The model under review builds one solid part; all positions refer to its coordinate system, in mm. Face numbers are marked on the shaded views. A direction names the side the tool comes from. Round coordinates to 2 decimals unless told otherwise and drop trailing zeros. Order: outer loops, then holes, each group sorted by start corner. A loop starts at its lowest first (then second) coordinate and runs counter-clockwise, first axis right, second up. Notation, with made-up numbers: M 42.25,-19 L 72.25,-19 A27 cw 72.25,15 Z; hole C -22,58.25 d3. An arc over 180 degrees is marked long. Answer as a JSON object with one key per item and string values. Group by question number.
1. To check wall thickness, follow probe 1 along X at (y, z) = (17, 34); probe 2 along X at (y, z) = (25, 36); probe 3 along X at (y, z) = (6, 5). State the ranges of each line that lie inside material, in increasing order. Write a range as [from, to].
2. Mouldability with a two-part tool opening along Y and no side actions: class the marked faces 6, 7 and 8 as released by +Y, released by -Y, zero draft, split by the parting line, or undercut.
3. Clearance check with flat-ended pins moving along their axes: P1, Ø19, axis at y = 50, z = 21, coming from the -X side; P2, Ø1.5, axis at y = 31, z = 18.5, coming from the -X side; P3, Ø2.5, axis at x = 38.5, z = 19.5, coming from the -Y side; P4, Ø21, axis at x = 58, y = 16, coming from the +Z side. State where each tip first meets the part, or that it passes through.
4. Machinability: for the marked faces 1, 2, 3, 4 and 5, which of the approach directions +Z, -Z, +X, -X, +Y, -Y give a long, thin tool a straight path to every point of the face, cutting with its end or side? Answer none if there is none.
5. Add section A-A on z = 24. Give the number of separate pieces and of enclosed holes in the cut face, and give its area (3 significant figures).
6. Add section D-D on x = 37. State the section outline as (y, z) points, and give its area (3 significant figures).
7. Add section B-B on y = 57.5. State the section outline as (x, z) points, and give its area (3 significant figures).
```python
from build123d import *

# Parameters (mm, degrees)
SKETCH1_W               = 74
SKETCH1_H               = 32
SKETCH1_R               = 11.7
BOSS_EXTRUDE1_DEPTH     = 38.5
SKETCH2_R               = 1.575
SKETCH2_R_2             = 10.75
BOSS_EXTRUDE2_DEPTH     = 5
BOSS_EXTRUDE3_DEPTH     = 5
CUT_EXTRUDE1_DEPTH      = 112.012668196
CUT_EXTRUDE1_DEPTH_BACK = 112.012668196
SKETCH4_W               = 10
SKETCH4_H               = 25
SKETCH4_H_2             = 4.450035805
SKETCH5_R               = 2.15
CUT_EXTRUDE2_DEPTH      = 18
FILLET8_R               = 16
FILLET9_R               = 1.5
FILLET10_SIZE           = 2
CUT_EXTRUDE3_DEPTH      = 3


with BuildPart() as part:
    # Sketch1 → Boss-Extrude1 (new body)
    with BuildSketch(Plane.XY):
        with Locations((37, 16)):
            Rectangle(SKETCH1_W, SKETCH1_H)
        with Locations((16, 16)):
            Circle(SKETCH1_R, mode=Mode.SUBTRACT)
        with Locations((58, 16)):
            Circle(SKETCH1_R, mode=Mode.SUBTRACT)
    extrude(amount=BOSS_EXTRUDE1_DEPTH)

    # Sketch2 → Boss-Extrude2 (add)
    # profile 1 of 2: a face of its own
    with BuildSketch(Plane(origin=(74, 0, 0), x_dir=(0, 0, -1), z_dir=(1, 0, 0))):
        with BuildLine():
            Line((-38.5, 32), (0, 32))
            Line((0, 32), (0, 54))
            ThreePointArc((0, 54), (-19.25, 34.75), (-38.5, 54))
            Line((-38.5, 54), (-38.5, 32))
        make_face()
    # profile 2 of 2: a face of its own
    with BuildSketch(Plane(origin=(74, 0, 0), x_dir=(0, 0, -1), z_dir=(1, 0, 0))):
        with BuildLine():
            ThreePointArc((-38.5, 54), (-19.25, 34.75), (0, 54))
            ThreePointArc((0, 54), (-19.25, 73.25), (-38.5, 54))
        make_face()
        with Locations((-28.249026536, 43.275377796)):
            Circle(SKETCH2_R, mode=Mode.SUBTRACT)
        with Locations((-24.038282007, 67.155696691)):
            Circle(SKETCH2_R, mode=Mode.SUBTRACT)
        with Locations((-19.25, 54)):
            Circle(SKETCH2_R_2, mode=Mode.SUBTRACT)
        with Locations((-5.462691458, 51.568925513)):
            Circle(SKETCH2_R, mode=Mode.SUBTRACT)
    extrude(amount=-BOSS_EXTRUDE2_DEPTH)

    # Sketch3 → Boss-Extrude3 (add)
    with BuildSketch(Plane.ZY.offset(-69)):
        with BuildLine():
            Line((0, 43), (0, 32))
            Line((0, 32), (38.5, 32))
            Line((38.5, 32), (38.5, 43))
            Line((38.5, 43), (36.548843892, 43))
            ThreePointArc((36.548843892, 43), (19.25, 33.5), (1.951156108, 43))
            Line((1.951156108, 43), (0, 43))
        make_face()
    extrude(amount=BOSS_EXTRUDE3_DEPTH)

    # Sketch4 → Cut-Extrude1 (cut, two sides: drawn at the far end of the back side and taken through both)
    with BuildSketch(Plane(origin=(0, 0, 0), x_dir=(-1, 0, 0), z_dir=(0, 0, -1)).offset(-CUT_EXTRUDE1_DEPTH_BACK)):
        with Locations((-37, 23.950035805)):
            Rectangle(SKETCH4_W, SKETCH4_H)
        with Locations((-37, 34.225017902)):
            Rectangle(SKETCH4_W, SKETCH4_H_2)
    extrude(amount=CUT_EXTRUDE1_DEPTH + CUT_EXTRUDE1_DEPTH_BACK, mode=Mode.SUBTRACT)

    # Sketch5 → Cut-Extrude2 (cut)
    with BuildSketch(Plane(origin=(0, 11.450035805, 0), x_dir=(1, 0, 0), z_dir=(0, 1, 0))):
        with Locations(Location((37, -19.25, 0), (0, 0, 270))):
            Circle(SKETCH5_R)
    extrude(amount=-CUT_EXTRUDE2_DEPTH, mode=Mode.SUBTRACT)

    # Fillet8
    fillet8_edges = [part.edges().sort_by_distance(p)[0] for p in [
        (42, 32, 19.25),
        (32, 32, 19.25),
        (0, 32, 19.25),
        (0, 0, 19.25),
        (74, 0, 19.25),
    ]]
    fillet(fillet8_edges, radius=FILLET8_R - 0.0001)  # a hair under: the kernel refuses the full size

    # Fillet9
    fillet9_edges = [part.edges().sort_by_distance(p)[0] for p in [
        (66.5, 43, 36.548843892),
        (66.5, 43, 1.951156108),
        (64, 32, 19.25),
    ]]
    fillet(fillet9_edges, radius=FILLET9_R - 0.0001)  # a hair under: the kernel refuses the full size

    # Fillet10
    fillet10_edges = [part.edges().sort_by_distance(p)[0] for p in [
        (4.3, 16, 0),
        (4.3, 16, 38.5),
        (46.3, 16, 0),
        (46.3, 16, 38.5),
    ]]
    chamfer(fillet10_edges, length=FILLET10_SIZE)

    # Sketch6 → Cut-Extrude3 (cut)
    with BuildSketch(Plane.XZ):
        Polygon((39.110229916, 15.468871901), (41.329667947, 19.186948665), (39.219438031, 22.968076764), (34.889770084, 23.031128099), (32.670332053, 19.313051335), (34.780561969, 15.531923236), align=None)
    extrude(amount=-CUT_EXTRUDE3_DEPTH, mode=Mode.SUBTRACT)


solid = part.part
```
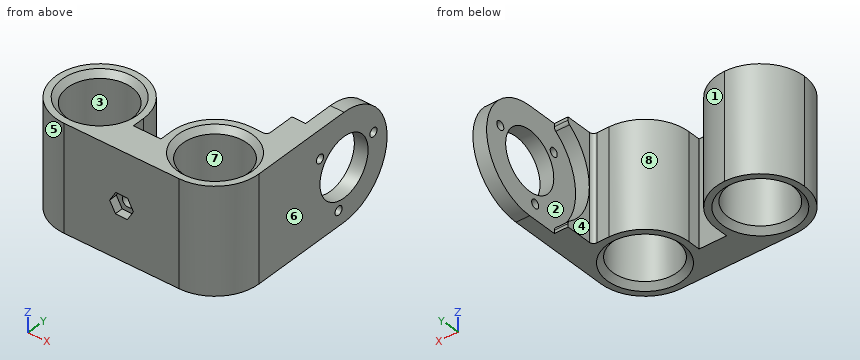
Recorded:
{
 "1": {"probe 1": "x = [0.03, 4.34], [27.66, 31.97], [42.03, 46.34], [69.66, 74]", "probe 2": "x = [2.77, 8.52], [23.48, 29.23], [44.77, 50.52], [65.48, 74]", "probe 3": "x = [3.51, 9.93], [22.07, 51.93], [64.07, 70.49]"},
 "2": {"face 6": "zero draft", "face 7": "undercut", "face 8": "released by +Y"},
 "3": {"P1": "stops at x = 69", "P2": "stops at x = 8.72", "P3": "stops at y = 3", "P4": "passes through"},
 "4": {"face 1": "+Z, -Z, +Y", "face 2": "-X, +Y", "face 3": "+Z, -Z", "face 4": "+Z, -Z, -X, +Y", "face 5": "+Z, -Z, -X, -Y"},
 "5": {"separate pieces": "3", "enclosed holes": "2", "area": "1,130 mm²"},
 "6": {"outline": "M 0,0 L 11.45,0 L 11.45,17.1 L 3,17.1 L 3,15.5 L 0,15.5 Z; M 0,23 L 3,23 L 3,21.4 L 11.45,21.4 L 11.45,38.5 L 0,38.5 Z", "area": "382 mm²"},
 "7": {"outline": "M 69,0.32 L 74,0.32 L 74,9.09 L 69,9.09 Z; M 69,29.41 L 74,29.41 L 74,38.18 L 69,38.18 Z", "area": "87.6 mm²"}
}
